Verification items for the finished model (mm, model axes). Face numbers are marked on the shaded views. A direction names the side the tool comes from. Round coordinates to 2 decimals unless told otherwise and drop trailing zeros. Write each loop counter-clockwise with the first axis right and the second up, starting at its lowest first coordinate (ties: lowest second). Pieces come first, ordered by that corner, then holes.
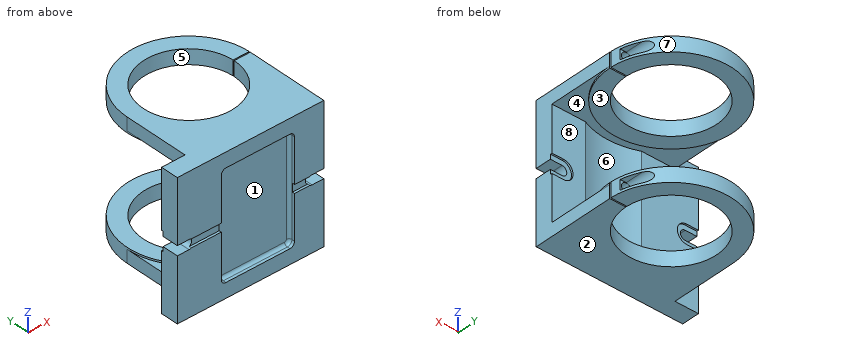
from build123d import *

# Parameters (mm, degrees)
SKETCH_2_W                 = 250
SKETCH_2_H                 = 230
EXTRUDE_1_DEPTH            = 30
CUT_EXTRUDE_1_DEPTH        = 3
CUT_EXTRUDE_2_DEPTH        = 188.026736057
CUT_EXTRUDE_3_DEPTH        = 10
FILLET_1_R                 = 5
SKETCH_6_W                 = 14
SKETCH_6_H                 = 8
CUT_EXTRUDE_4_DEPTH        = 277.812210713
SKETCH_7_R                 = 77.5
EXTRUDE_2_DEPTH            = 25
CUT_EXTRUDE_1_2_DEPTH      = 308.042342357
CUT_EXTRUDE_1_2_DEPTH_BACK = 308.042342357
SKETCH_8_W                 = 153.899728908
SKETCH_8_H                 = 2
SKETCH_9_R                 = 8
CUT_EXTRUDE_5_DEPTH        = 16
CUT_EXTRUDE_6_DEPTH        = 244.339269334
CUT_EXTRUDE_START          = -3
CUT_EXTRUDE_7_DEPTH        = 186


with BuildPart() as part:
    # 草图2 → 凸台-拉伸1 (new body)
    with BuildSketch(Plane(origin=(0, 0, 0), x_dir=(1, 0, 0), z_dir=(0, 1, 0))):
        with Locations((-20, 0)):
            Rectangle(SKETCH_2_W, SKETCH_2_H)
    extrude(amount=EXTRUDE_1_DEPTH)

    # 草图3 → Cut-Extrude 1 (cut)
    with BuildSketch(Plane(origin=(0, 30, 0), x_dir=(1, 0, 0), z_dir=(0, 1, 0))):
        with BuildLine():
            Line((-145, 16), (-125, 16))
            ThreePointArc((-125, 16), (-109, 0), (-125, -16))
            Line((-125, -16), (-145, -16))
            ThreePointArc((-145, -16), (-161, 0), (-145, 16))
        make_face()
    cut_extrude_1 = extrude(amount=-CUT_EXTRUDE_1_DEPTH, mode=Mode.SUBTRACT)

    # 草图4 → 切除-拉伸2 (cut, through all)
    with BuildSketch(Plane(origin=(0, 27, 0), x_dir=(1, 0, 0), z_dir=(0, 1, 0))):
        with BuildLine():
            Line((-145, 8), (-145, -8))
            Line((-145, -8), (-125, -8))
            ThreePointArc((-125, -8), (-117, 0), (-125, 8))
            Line((-125, 8), (-145, 8))
        make_face()
    cut_extrude_2 = extrude(amount=-CUT_EXTRUDE_2_DEPTH, mode=Mode.SUBTRACT)

    # 镜向1: Cut-Extrude 1, 切除-拉伸2 across plane
    add(cut_extrude_1.mirror(Plane.ZY.offset(20)), mode=Mode.SUBTRACT)
    add(cut_extrude_2.mirror(Plane.ZY.offset(20)), mode=Mode.SUBTRACT)

    # 草图5 → 切除-拉伸3 (cut)
    with BuildSketch(Plane.XZ):
        with BuildLine():
            Line((-62, -90), (47, -90))
            ThreePointArc((47, -90), (52.656854249, -87.656854249), (55, -82))
            Line((55, -82), (55, 82))
            ThreePointArc((55, 82), (52.656854249, 87.656854249), (47, 90))
            Line((47, 90), (-62, 90))
            ThreePointArc((-62, 90), (-67.656854249, 87.656854249), (-70, 82))
            Line((-70, 82), (-70, -82))
            ThreePointArc((-70, -82), (-67.656854249, -87.656854249), (-62, -90))
        make_face()
    extrude(amount=-CUT_EXTRUDE_3_DEPTH, mode=Mode.SUBTRACT)

    # 圆角1
    fillet_1_edges = [part.edges().sort_by_distance(p)[0] for p in [
        (52.656854249, 10, -87.656854249),
        (-7.5, 10, -90),
        (-67.656854249, 10, -87.656854249),
        (-70, 10, 0),
        (-67.656854249, 10, 87.656854249),
        (-7.5, 10, 90),
        (52.656854249, 10, 87.656854249),
        (55, 10, 0),
    ]]
    fillet(fillet_1_edges, radius=FILLET_1_R)

    # 草图6 → 切除-拉伸4 (cut, through all)
    with BuildSketch(Plane.ZY.offset(145)):
        Rectangle(SKETCH_6_W, SKETCH_6_H)
    extrude(amount=-CUT_EXTRUDE_4_DEPTH, mode=Mode.SUBTRACT)

    # 草图7 → 凸台-拉伸2 (add)
    with BuildSketch(Plane.XY.offset(115)):
        with BuildLine():
            Line((105, 30), (105, 140))
            ThreePointArc((105, 140), (0, 245), (-105, 140))
            Line((-105, 140), (-105, 30))
            Line((-105, 30), (105, 30))
        make_face()
        with Locations((0, 140)):
            Circle(SKETCH_7_R, mode=Mode.SUBTRACT)
    extrude_2 = extrude(amount=-EXTRUDE_2_DEPTH)

    # 镜向2: 凸台-拉伸2 across plane
    add(extrude_2.mirror(Plane.XY))

    # 草图8 → Cut-Extrude 1 2 (cut, two sides: drawn at the far end of the back side and taken through both)
    with BuildSketch(Plane.XY.offset(-CUT_EXTRUDE_1_2_DEPTH_BACK)):
        with Locations((76.949864454, 141)):
            Rectangle(SKETCH_8_W, SKETCH_8_H)
    extrude(amount=CUT_EXTRUDE_1_2_DEPTH + CUT_EXTRUDE_1_2_DEPTH_BACK, mode=Mode.SUBTRACT)

    # 草图9 → 切除-拉伸5 (cut)
    with BuildSketch(Plane.XZ.offset(-142)):
        with Locations(Location((93, 102.5, 0), (0, 0, 270))):
            Circle(SKETCH_9_R)
    cut_extrude_5 = extrude(amount=-CUT_EXTRUDE_5_DEPTH, mode=Mode.SUBTRACT)

    # 草图10 → 切除-拉伸6 (cut, through all)
    with BuildSketch(Plane.XZ.offset(-158)):
        with BuildLine():
            Line((93, 111), (105, 111))
            Line((105, 111), (105, 94))
            Line((105, 94), (93, 94))
            ThreePointArc((93, 94), (84.5, 102.5), (93, 111))
        make_face()
    cut_extrude_6 = extrude(amount=-CUT_EXTRUDE_6_DEPTH, mode=Mode.SUBTRACT)

    # 草图12 → M10 螺纹孔1 (revolve, cut)
    with BuildSketch(Plane(origin=(93, 140, 102.5), x_dir=(0, 0, 1), z_dir=(1, 0, 0))):
        Polygon((0, 0), (0, 32.553657631), (4.25, 30), (4.25, 0), align=None)
    hole_wizard_m10_1 = revolve(axis=Axis((93, 146.35, 102.5), (0, -1, 0)), mode=Mode.SUBTRACT)

    # 镜向3: 切除-拉伸5, 切除-拉伸6, M10 螺纹孔1 across plane
    add(cut_extrude_5.mirror(Plane.XY), mode=Mode.SUBTRACT)
    add(cut_extrude_6.mirror(Plane.XY), mode=Mode.SUBTRACT)
    add(hole_wizard_m10_1.mirror(Plane.XY), mode=Mode.SUBTRACT)

    # 草图13 → 切除-拉伸7 (cut)
    with BuildSketch(Plane.XY.offset(-90).offset(CUT_EXTRUDE_START)):
        with BuildLine():
            Line((47.958315233, 30), (105, 30))
            Line((105, 30), (105, 140))
            ThreePointArc((105, 140), (0, 35), (-105, 140))
            Line((-105, 140), (-105, 30))
            Line((-105, 30), (-47.958315233, 30))
            ThreePointArc((-47.958315233, 30), (0, 20), (47.958315233, 30))
        make_face()
    extrude(amount=CUT_EXTRUDE_7_DEPTH, mode=Mode.SUBTRACT)


solid = part.part
Q1. Sectioned sample at A-A (x = 0). Enter the section's corners in (y, z).
Recorded:
outline: (0, -115) - (62.5, -115) - (62.5, -90) - (35, -90) - (35, -93) - (20, -93) - (20, 93) - (35, 93) - (35, 90) - (62.5, 90) - (62.5, 115) - (0, 115) - (0, 90) - (5, 90) arc R5 cw to (10, 85) - (10, -85) arc R5 cw to (5, -90) - (0, -90) - close; (217.5, -115) - (245, -115) - (245, -90) - (217.5, -90) - close; (217.5, 90) - (245, 90) - (245, 115) - (217.5, 115) - close
Q2. Sectioned sample at D-D (y = 74). Enter the section's corners in (x, z), plus the area to 3 significant figures.
Recorded:
outline: (-105, -115) - (-40.62, -115) - (-40.62, -90) - (-81.66, -90) - (-81.66, -93) - (-105, -93) - close; (-105, 93) - (-81.66, 93) - (-81.66, 90) - (-40.62, 90) - (-40.62, 115) - (-105, 115) - close; (40.62, -115) - (105, -115) - (105, -93) - (81.66, -93) - (81.66, -90) - (40.62, -90) - close; (40.62, 90) - (81.66, 90) - (81.66, 93) - (105, 93) - (105, 115) - (40.62, 115) - close
area: 6,160 mm2
Q3. Sectioned sample at B-B (y = 124). Enter the section's corners in (x, z).
Recorded:
outline: (-105, -115) - (-75.83, -115) - (-75.83, -90) - (-103.77, -90) - (-103.77, -93) - (-105, -93) - close; (-105, 93) - (-103.77, 93) - (-103.77, 90) - (-75.83, 90) - (-75.83, 115) - (-105, 115) - close; (75.83, -115) - (105, -115) - (105, -93) - (103.77, -93) - (103.77, -90) - (75.83, -90) - close; (75.83, 90) - (103.77, 90) - (103.77, 93) - (105, 93) - (105, 115) - (75.83, 115) - close; hole circle Ø8.5 at (93, -102.5); hole circle Ø8.5 at (93, 102.5)
Q4. Material ranges on line 1 along Z through (x, y) = (93, 132.25); line 2 along Z through (x, y) = (90, 175.5); line 3 along Z through (x, y) = (-70, 38.5), recorded low to high.
Recorded:
line 1: z = -115 to -106.75, -98.25 to -90, 90 to 98.25, 106.75 to 115
line 2: z = -115 to -110.45, -94.55 to -90, 90 to 94.55, 110.45 to 115
line 3: z = -115 to -93, 93 to 115
Q5. Tool access check on the marked faces 1, 2, 3 and 4. Record the directions out of +Z, -Z, +X, -X, +Y, -Y that give a thin tool (end or side, any length) a straight path to the whole face; none if there is none.
Recorded:
face 1: -Y
face 2: -Z, +X, -X, +Y, -Y
face 3: +X, -X, +Y
face 4: none
Q6. Release check for a two-part mould opening along X. For the marked faces 5, 6, 7 and 8 record: released by +X, released by -X, zero draft, split by the parting line, or undercut.
Recorded:
face 5: undercut
face 6: undercut
face 7: split by the parting line
face 8: zero draft
Q7. Sectioned sample at C-C (z = 0). Enter the section's corners in (x, y), plus the area to 3 significant figures.
Recorded:
outline: (-117, 4) - (-70, 4) - (-70, 5) arc R5 cw to (-65, 10) - (50, 10) arc R5 cw to (55, 5) - (55, 4) - (77, 4) - (77, 27) - (69, 27) - (69, 30) - (47.96, 30) arc R120 cw to (-47.96, 30) - (-109, 30) - (-109, 27) - (-117, 27) - close
area: 3,610 mm2
Q8. Depth check by flat-ended pin: P1, Ø8.5, axis at x = 93.5, z = -106, coming from the +Y side; P2, Ø24, axis at y = 82, z = 102, coming from the -X side; P3, Ø1.5, axis at x = -85, z = -1, coming from the -Y side. Enter the tip coordinate at first touch or a pass-through.
Recorded:
P1: stops at y = 140
P2: stops at x = -105
P3: stops at y = 4
